```python
from build123d import *

# Parameters (mm, degrees)
EXTRUDE_1_DEPTH      = 10
EXTRUDE_2_DEPTH      = 10
EXTRUDE_2_DEPTH_BACK = 10
SKETCH_2_W           = 20
SKETCH_2_H           = 4
SKETCH_3_R           = 1.5
CUT_EXTRUDE_1_DEPTH  = 10
SKETCH_4_R           = 1.5
CUT_EXTRUDE_2_DEPTH  = 10


with BuildPart() as part:
    # 草图1 → 凸台-拉伸1 (new body)
    with BuildSketch(Plane.XY):
        Polygon((0, 0), (12, 0), (12, 4), (7, 4), (7, 7.071067812), (-21.213203436, 35.284271247), (-24.748737342, 31.748737342), (0, 7), align=None)
    extrude(amount=EXTRUDE_1_DEPTH)

    # 草图2 → 凸台-拉伸2 (add, two sides: drawn at the far end of the back side and taken through both)
    with BuildSketch(Plane(origin=(0, 0, 0), x_dir=(-1, 0, 0), z_dir=(0, 0, -1)).offset(-EXTRUDE_2_DEPTH_BACK)):
        with Locations((-2, 2)):
            Rectangle(SKETCH_2_W, SKETCH_2_H)
    extrude(amount=EXTRUDE_2_DEPTH + EXTRUDE_2_DEPTH_BACK)

    # 草图3 → 切除-拉伸1 (cut)
    with BuildSketch(Plane(origin=(7.035533906, 7.035533906, 0), x_dir=(0, 0, -1), z_dir=(0.7071067811865465, 0.7071067811865486, 0))):
        with Locations(Location((-5, 17.949747468, 0), (0, 0, 90))):
            Circle(SKETCH_3_R)
    extrude(amount=-CUT_EXTRUDE_1_DEPTH, mode=Mode.SUBTRACT)

    # 草图4 → 切除-拉伸2 (cut)
    with BuildSketch(Plane(origin=(0, 4, 0), x_dir=(1, 0, 0), z_dir=(0, 1, 0))):
        with Locations(Location((-5, 5, 0), (0, 0, 180))):
            Circle(SKETCH_4_R)
        with Locations(Location((3, 5, 0), (0, 0, 180))):
            Circle(SKETCH_4_R)
    extrude(amount=-CUT_EXTRUDE_2_DEPTH, mode=Mode.SUBTRACT)


solid = part.part
```
Geometry check sheet. Reference: the model listing, model coordinates, mm. A direction names the side the tool comes from. Give positions to 0.01 mm unless a question says otherwise; leave off trailing zeros. Write each loop counter-clockwise with the first axis right and the second up, starting at its lowest first coordinate (ties: lowest second). Pieces come first, ordered by that corner, then holes. Notation, with made-up numbers: (37, 47) - (71, 47) arc R24 cw to (71, 61) - close; hole circle Ø2 at (24, 72.25). An arc over 180 degrees is marked (long way). Use a Markdown table: item, result.
Q1. Section check C-C, the plane z = 5.5. Enter the section's corners in (x, y).
Computed:
| item | result |
|---|---|
| outline | (-24.75, 31.75) - (-10.19, 17.19) - (-6.66, 20.73) - (-21.21, 35.28) - close; (-8.19, 15.19) - (0, 7) - (0, 4) - (-8, 4) - (-8, 0) - (12, 0) - (12, 4) - (7, 4) - (7, 7.07) - (-4.66, 18.73) - close |
Q2. Set-up check for faces 1 (the face through (7, 6, 5)), 2 (the face through (0, 6, 5)), 3 (the face through (2, 4, -2)), 4 (the face through (-23, 33.5, 4.9)): record each of +Z, -Z, +X, -X, +Y, -Y from which the full face is reachable in a straight line by a thin tool's end or side.
Computed:
| item | result |
|---|---|
| face 1 | +Z, -Z, +X, +Y |
| face 2 | +Z, -Z, -X |
| face 3 | -Z |
| face 4 | +Z, -Z, -X, +Y |
Q3. Section check D-D, the plane x = -4. Enter the section's corners in (y, z), then the cut area to 3 significant figures.
Computed:
| item | result |
|---|---|
| outline | (0, -10) - (4, -10) - (4, -6.12) - (0, -6.12) - close; (0, -3.88) - (4, -3.88) - (4, 10) - (0, 10) - close; (11, 0) - (18.07, 0) - (18.07, 10) - (11, 10) - close |
| area | 142 mm² |
Q4. Thickness scan on L1, parallel to Z at x = -5, y = 1; L2, parallel to Z at x = -10.5, y = 21; L3, parallel to Y at x = 0.5, z = -0.5. Record the ranges inside material, lowest first. Write a range as [from, to].
Computed:
| item | result |
|---|---|
| L1 | z = [-10, -6.5], [-3.5, 10] |
| L2 | z = [0, 10] |
| L3 | y = [0, 4] |
Q5. Draft check along Z on faces 5 (the face through (-9, 19, 0)), 6 (the face through (1.57, 2.03, -4.55)), 7 (the face through (-8, 2, 0)). Enter one of: pulls with the +Z half, pulls with the -Z half, needs draft (parallel to the pull), parting line crosses it, or undercut.
Computed:
| item | result |
|---|---|
| face 5 | pulls with the -Z half |
| face 6 | undercut |
| face 7 | needs draft |
Q6. Section check A-A, the plane z = -5. Enter the section's corners in (x, y), then the cut area to 3 significant figures.
Computed:
| item | result |
|---|---|
| outline | (-8, 0) - (-6.5, 0) - (-6.5, 4) - (-8, 4) - close; (-3.5, 0) - (1.5, 0) - (1.5, 4) - (-3.5, 4) - close; (4.5, 0) - (12, 0) - (12, 4) - (4.5, 4) - close |
| area | 56.0 mm² |
Q7. Go/stop test with flat-tipped pins: P1, Ø1.5, axis at y = 5, z = 3, coming from the +X side; P2, Ø2.5, axis at x = -5, z = -5, coming from the -Y side; P3, Ø3, axis at y = 13.5, z = 5.5, coming from the +X side; P4, Ø5, axis at x = 3, z = -5, coming from the +Y side. Record where each tip stops, or that it passes through.
Computed:
| item | result |
|---|---|
| P1 | stops at x = 7 |
| P2 | passes through |
| P3 | stops at x = 2.07 |
| P4 | stops at y = 4 |
Q8. Section check B-B, the plane x = 3. Enter the section's corners in (y, z).
Computed:
| item | result |
|---|---|
| outline | (0, -10) - (4, -10) - (4, -6.5) - (0, -6.5) - close; (0, -3.5) - (4, -3.5) - (4, 0) - (11.07, 0) - (11.07, 10) - (0, 10) - close |
